Source: CAD feature listing. Evaluate the final solid. Frame: model axes, mm. A direction names the side the tool comes from. Round coordinates to 2 decimals unless told otherwise and drop trailing zeros. Loops run counter-clockwise (first coordinate to the right, second up) from the corner with the lowest first, then second, coordinate; pieces in that order, holes last.
Item 1: Section query B-B on y = 153. Return loops of the section in (x, z), then the cut area to 3 significant figures.
Item 2: Ray query, L1, parallel to Y at x = -45, z = 4.55; L2, parallel to Y at x = 35, z = 1.35; L3, parallel to X at y = 382.5, z = 3.6. Return the intervals inside material, ascending.
Item 3: First-contact query: P1, Ø1.4, axis at x = 30.5, z = 2.5, coming from the +Y side; P2, Ø2, axis at y = 340, z = 4, coming from the -X side; P3, Ø2, axis at y = 169, z = 3, coming from the +X side. Flat tips, straight axial feed; report the tip coordinate or a pass-through.
Item 4: Pull-direction query (X, two-part tool) for faces 1 (the flat face through (214.2, 143.31, 2.41)), 2 (the flat face through (156.808, 344.318, 2.348)), 3 (the flat face through (-311.23, 55.13, 2.35)); classes: released by +X, released by -X, zero draft, split by the parting line, or undercut.
Item 5: Section query A-A on x = -14.5. Return loops of the section in (y, z).
Item 6: Section query C-C on z = 2.2. Give the number of separate pieces and of enclosed holes in the cut face, then the cut area to 3 significant figures.
Item 7: Access query for faces 4 (the cylindrical face through (-147.49, 247.41, 2.41)), 5 (the flat face through (267.41, 152.75, 2.35)). Directions: +Z, -Z, +X, -X, +Y, -Y. A direction counts if a zero-diameter tool reaches every point of the face in a straight line with its end or side. Return the directions, or none.
```python
from build123d import *

# Parameters (mm, degrees)
BOSS_EXTRUDE1_DEPTH = 4.7625
CUT_EXTRUDE5_DEPTH  = 515.11412225
CUT_EXTRUDE15_DEPTH = 4.7625
FILLET1_R           = 19.05
CUT_EXTRUDE9_DEPTH  = 515.11412225
CUT_EXTRUDE10_DEPTH = 515.11412225
SKETCH4_W           = 50.8
SKETCH4_H           = 4.7625
CUT_EXTRUDE11_DEPTH = 515.11412225
SKETCH14_W          = 12.7
SKETCH14_H          = 25.4
CUT_EXTRUDE12_DEPTH = 515.11412225
CUT_EXTRUDE13_REACH = 516.114
CUT_EXTRUDE14_REACH = 516.114
MIRROR1_DEPTH       = 4.7625


# Read off the part's stored shape, not the designer's step: Mirror1
with BuildPart() as part:
    # Sketch3 → Boss-Extrude1 (new body)
    with BuildSketch(Plane.XY):
        Polygon((-317.5, 65.991135768), (-279.4, 0), (279.4, 0), (317.5, 65.991135768), (122.15878735, 404.332040891), (-122.15878735, 404.332040891), align=None)
    extrude(amount=BOSS_EXTRUDE1_DEPTH)

    # Sketch7 → Cut-Extrude5 (cut, through all)
    with BuildSketch(Plane.XY.offset(4.7625)):
        with BuildLine():
            Line((-136.142811828, 240.411), (136.142811828, 240.411))
            ThreePointArc((136.142811828, 240.411), (147.405476624, 247.242236784), (146.551931965, 260.387002884))
            Line((146.551931965, 260.387002884), (94.11202324, 335.408043775))
            ThreePointArc((94.11202324, 335.408043775), (89.571666319, 339.394705687), (83.702903103, 340.832040891))
            Line((83.702903103, 340.832040891), (-83.702903103, 340.832040891))
            ThreePointArc((-83.702903103, 340.832040891), (-89.571666319, 339.394705687), (-94.11202324, 335.408043775))
            Line((-94.11202324, 335.408043775), (-146.551931965, 260.387002884))
            ThreePointArc((-146.551931965, 260.387002884), (-147.405476624, 247.242236784), (-136.142811828, 240.411))
        make_face()
    extrude(amount=-CUT_EXTRUDE5_DEPTH, mode=Mode.SUBTRACT)

    # Sketch11 → Cut-Extrude15 (cut)
    with BuildSketch(Plane.XY.offset(4.7625)):
        Polygon((-172.804553922, 215.011), (172.804553922, 215.011), (267.611818975, 50.8), (-267.611818975, 50.8), align=None)
    extrude(amount=-CUT_EXTRUDE15_DEPTH, mode=Mode.SUBTRACT)

    # Fillet1
    fillet1_edges = [part.edges().sort_by_distance(p)[0] for p in [
        (172.804553922, 215.011, 2.38125),
        (-172.804553922, 215.011, 2.38125),
        (-267.611818975, 50.8, 2.38125),
        (267.611818975, 50.8, 2.38125),
    ]]
    fillet(fillet1_edges, radius=FILLET1_R)

    # Sketch12 → Cut-Extrude9 (cut, through all)
    with BuildSketch(Plane.XY.offset(4.7625)):
        Polygon((215.9, 241.967497817), (190.5, 285.96158833), (187.750369343, 284.37408833), (213.150369343, 240.379997817), align=None)
        Polygon((-187.750369343, 284.37408833), (-213.150369343, 240.379997817), (-215.9, 241.967497817), (-190.5, 285.96158833), align=None)
    extrude(amount=-CUT_EXTRUDE9_DEPTH, mode=Mode.SUBTRACT)

    # Sketch13 → Cut-Extrude10 (cut, through all)
    with BuildSketch(Plane.XY.offset(4.7625)):
        Polygon((292.077815329, 21.958620278), (287.953369343, 24.339870278), (300.653369343, 46.336915534), (304.777815329, 43.955665534), align=None)
        Polygon((-300.653369343, 46.336915534), (-304.777815329, 43.955665534), (-292.077815329, 21.958620278), (-287.953369343, 24.339870278), align=None)
    extrude(amount=-CUT_EXTRUDE10_DEPTH, mode=Mode.SUBTRACT)

    # Sketch4 → Cut-Extrude11 (cut, through all)
    with BuildSketch(Plane.XY.offset(4.7625)):
        with Locations((200.450369343, 2.38125)):
            Rectangle(SKETCH4_W, SKETCH4_H)
        with Locations((-200.450369343, 2.38125)):
            Rectangle(SKETCH4_W, SKETCH4_H)
    extrude(amount=-CUT_EXTRUDE11_DEPTH, mode=Mode.SUBTRACT)

    # Sketch14 → Cut-Extrude12 (cut, through all)
    with BuildSketch(Plane.XY.offset(4.7625)):
        with Locations((-31.75, 391.632040891)):
            Rectangle(SKETCH14_W, SKETCH14_H)
        with Locations((31.75, 391.632040891)):
            Rectangle(SKETCH14_W, SKETCH14_H)
    extrude(amount=-CUT_EXTRUDE12_DEPTH, mode=Mode.SUBTRACT)

    # Sketch15 → Cut-Extrude13 (cut, up to next)
    with BuildSketch(Plane.XY.offset(4.7625), mode=Mode.PRIVATE) as cut_extrude13_sk1:
        Polygon((-281.426680084, 3.510312876), (-274.663389205, 0), (-268.812867745, 11.272151465), (-275.576158624, 14.782464341), align=None)
    cut_extrude13_tool1 = extrude(cut_extrude13_sk1.sketch, amount=-CUT_EXTRUDE13_REACH, mode=Mode.PRIVATE) & part.part
    add(cut_extrude13_tool1.solids().sort_by_distance((-275.119774, 7.391232, 4.7625))[0], mode=Mode.SUBTRACT)


with BuildPart() as cut_extrude13_kept_piece:
    # of the separate pieces the step leaves, the one the design keeps (cut_extrude13_pieces_kept)
    add(part.part.solids().sort_by_distance((-122.15878735, 404.332040891, 0))[0])

    # Sketch16 → Cut-Extrude14 (cut, up to next)
    with BuildSketch(Plane.XY.offset(4.7625), mode=Mode.PRIVATE) as cut_extrude14_sk1:
        Polygon((-187.750369343, 284.37408833), (-191.560369343, 277.774974753), (-184.961255766, 273.964974753), (-181.151255766, 280.56408833), align=None)
    cut_extrude14_tool1 = extrude(cut_extrude14_sk1.sketch, amount=-CUT_EXTRUDE14_REACH, mode=Mode.PRIVATE) & cut_extrude13_kept_piece.part
    add(cut_extrude14_tool1.solids().sort_by_distance((-186.355813, 279.169532, 4.7625))[0], mode=Mode.SUBTRACT)

    # Mirror1 outline → Mirror1 (cut)
    with BuildSketch(Plane.XY):
        Polygon((191.560369343, 277.774974753), (187.750369343, 284.37408833), (181.151255766, 280.56408833), (184.961255766, 273.964974753), align=None)
        Polygon((281.426680084, 3.510312876), (275.576158624, 14.782464341), (268.812867745, 11.272151465), (274.663389205, 0), (279.4, 0), align=None)
    extrude(amount=MIRROR1_DEPTH, mode=Mode.SUBTRACT)


solid = cut_extrude13_kept_piece.part
```
Data:
1. outline: (-267.27, 0) - (-208.61, 0) - (-208.61, 4.76) - (-267.27, 4.76) - close; (208.61, 0) - (267.27, 0) - (267.27, 4.76) - (208.61, 4.76) - close
1. area: 559 mm2
2. L1: y = 0 to 50.8, 215.01 to 240.41, 340.83 to 404.33
2. L2: y = 0 to 50.8, 215.01 to 240.41, 340.83 to 378.93
2. L3: x = -134.76 to -38.1, -25.4 to 25.4, 38.1 to 134.76
3. P1: stops at y = 378.93
3. P2: stops at x = -159.88
3. P3: stops at x = 258.61
4. face 1: undercut
4. face 2: released by +X
4. face 3: released by -X
5. outline: (0, 0) - (50.8, 0) - (50.8, 4.76) - (0, 4.76) - close; (215.01, 0) - (240.41, 0) - (240.41, 4.76) - (215.01, 4.76) - close; (340.83, 0) - (404.33, 0) - (404.33, 4.76) - (340.83, 4.76) - close
6. separate pieces: 1
6. enclosed holes: 2
6. area: 89,400 mm2
7. face 4: +Z, -Z
7. face 5: +Z, -Z, +X, +Y
